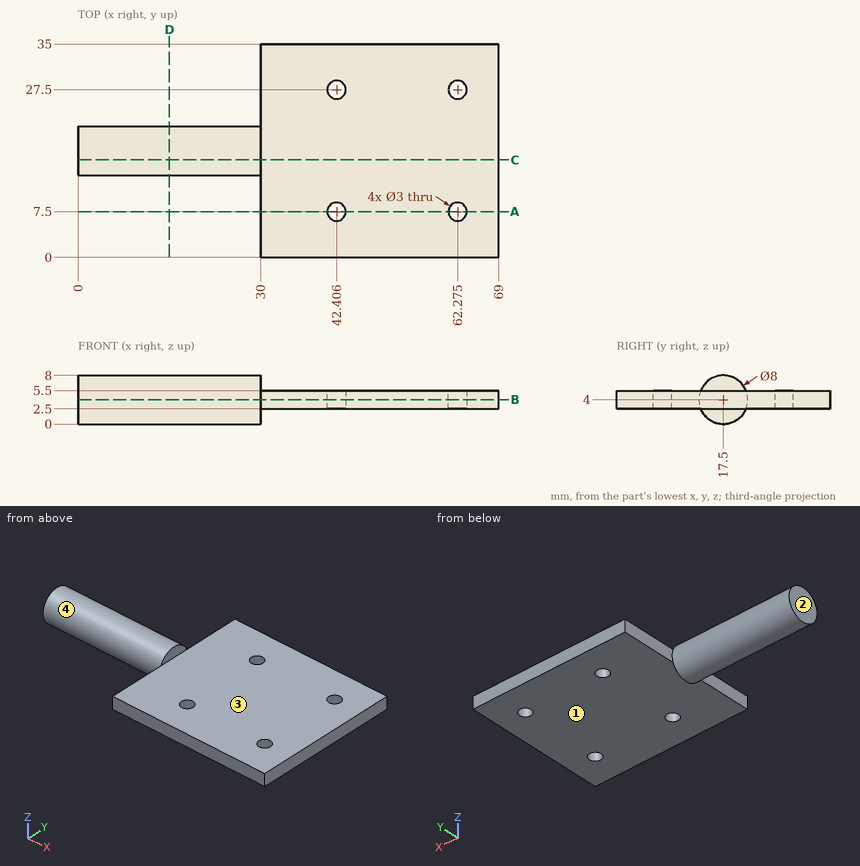
Design review of the part shown in the three views and the two pictorial views. Dimensions are in mm from the part's minimum x, y and z. A direction names the side the tool comes from. Give positions to 0.01 mm unless a question says otherwise; leave off trailing zeros. Loops run counter-clockwise (first coordinate to the right, second up) from the corner with the lowest first, then second, coordinate; pieces in that order, holes last. Notation, with made-up numbers: M 18,-19 L 76,-19 A34 cw 76,17 Z; hole C 67.25,46 d8. An arc over 180 degrees is marked long. Answer as a JSON object with one key per item and string values.
Item 1: For P1, Ø2, axis at y = 19, z = 0.5, coming from the +X side; P2, Ø3.5, axis at y = 28.5, z = 4.5, coming from the -X side; P3, Ø17.5, axis at x = 48, y = 11.5, coming from the +Z side; P4, Ø2.5, axis at x = 42.41, y = 27.5, coming from the +Z side, all flat-tipped, find the tip position at first contact; note any pin that passes through.
Output values:
{"P1": "stops at x = 30", "P2": "stops at x = 30", "P3": "stops at z = 5.5", "P4": "passes through"}
Item 2: Machinability: for the marked faces 1, 2, 3 and 4, which of the approach directions +Z, -Z, +X, -X, +Y, -Y give a long, thin tool a straight path to every point of the face, cutting with its end or side? Answer none if there is none.
Output values:
{"face 1": "-Z, +X, +Y, -Y", "face 2": "+Z, -Z, -X, +Y, -Y", "face 3": "+Z, +X, +Y, -Y", "face 4": "-X"}
Item 3: We need section C-C (y = 16). State the section outline as (x, z) points.
Output values:
{"outline": "M 0,0.29 L 30,0.29 L 30,2.5 L 69,2.5 L 69,5.5 L 30,5.5 L 30,7.71 L 0,7.71 Z"}
Item 4: We need section A-A (y = 7.5). State the section outline as (x, z) points (1 decimal).
Output values:
{"outline": "M 30,2.5 L 40.9,2.5 L 40.9,5.5 L 30,5.5 Z; M 43.9,2.5 L 60.8,2.5 L 60.8,5.5 L 43.9,5.5 Z; M 63.8,2.5 L 69,2.5 L 69,5.5 L 63.8,5.5 Z"}
Item 5: We need section B-B (z = 4). State the section outline as (x, y) points (1 decimal), and give its area (3 significant figures).
Output values:
{"outline": "M 0,13.5 L 30,13.5 L 30,0 L 69,0 L 69,35 L 30,35 L 30,21.5 L 0,21.5 Z; hole C 42.4,7.5 d3; hole C 42.4,27.5 d3; hole C 62.3,7.5 d3; hole C 62.3,27.5 d3", "area": "1,580 mm2"}
Item 6: Wall thickness on line 1 along Z through (x, y) = (58.5, 14.5); line 2 along Y through (x, z) = (17, 3.75); line 3 along X through (y, z) = (2, 3.5): over which ranges is each line inside the solid? List them lowest first.
Output values:
{"line 1": "z = 2.5 to 5.5", "line 2": "y = 13.51 to 21.49", "line 3": "x = 30 to 69"}
Item 7: We need section D-D (x = 15). State the section outline as (y, z) points.
Output values:
{"outline": "C 17.5,4 d8"}
